The listing builds one solid part. Answer for the finished solid, in the listing's coordinates (mm). Face numbers are marked on the shaded views. A direction names the side the tool comes from. Coordinates: 2 decimals unless noted, no trailing zeros. Write each loop counter-clockwise with the first axis right and the second up, starting at its lowest first coordinate (ties: lowest second). Pieces come first, ordered by that corner, then holes.
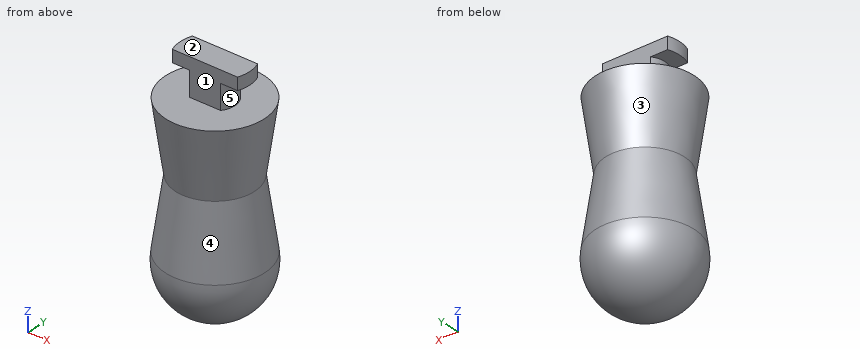
from build123d import *

# Parameters (mm, degrees)
F3_DEPTH = 9.525


with BuildPart() as f1:
    # F0 (on Front) → F1 (revolve)
    with BuildSketch(Plane.XZ):
        Polygon((0, -18.0305813839), (0, 0), (-5.08, 0), (-12.7, 0), (-10.16, -18.0305813839), align=None)
        Polygon((-5.08, 0), (0, 0), (0, 9.525), (-8.89, 9.525), (-8.89, 6.35), (-5.08, 6.35), align=None)
        Polygon((0, -36.0611627679), (0, -18.0305813839), (-10.16, -18.0305813839), (-12.7635, -36.0611627679), align=None)
        with BuildLine():
            Line((0, -50.8), (0, -36.0611627679))
            Line((0, -36.0611627679), (-12.7635, -36.0611627679))
            ThreePointArc((-12.7635, -36.0611627679), (-9.7485929139, -46.3461912692), (0, -50.8))
        make_face()
    revolve(axis=Axis((0, 0, -25.4), (0, 0, -1)))

    # F2 (on face) → F3 (cut, through all)
    with BuildSketch(Plane.XY.offset(9.525)):
        with BuildLine():
            ThreePointArc((8.3037024874, 3.175), (0, 8.89), (-8.3037024874, 3.175))
            Line((-8.3037024874, 3.175), (8.3037024874, 3.175))
        make_face()
        with BuildLine():
            Line((8.3037024874, -3.175), (-8.3037024874, -3.175))
            ThreePointArc((-8.3037024874, -3.175), (0, -8.89), (8.3037024874, -3.175))
        make_face()
        with BuildLine():
            ThreePointArc((10.9695693512, 3.175), (0, 11.4198107144), (-10.9695693512, 3.175))
            Line((-10.9695693512, 3.175), (-8.3037024874, 3.175))
            ThreePointArc((-8.3037024874, 3.175), (0, 8.89), (8.3037024874, 3.175))
            Line((8.3037024874, 3.175), (10.9695693512, 3.175))
        make_face()
        with BuildLine():
            Line((-8.3037024874, -3.175), (-10.9695693512, -3.175))
            ThreePointArc((-10.9695693512, -3.175), (0, -11.4198107144), (10.9695693512, -3.175))
            Line((10.9695693512, -3.175), (8.3037024874, -3.175))
            ThreePointArc((8.3037024874, -3.175), (0, -8.89), (-8.3037024874, -3.175))
        make_face()
        with BuildLine():
            Line((-8.3037024874, 3.175), (-10.9695693512, 3.175))
            ThreePointArc((-10.9695693512, 3.175), (-11.4198107144, 0), (-10.9695693512, -3.175))
            Line((-10.9695693512, -3.175), (-8.3037024874, -3.175))
            ThreePointArc((-8.3037024874, -3.175), (-8.89, 0), (-8.3037024874, 3.175))
        make_face()
        with BuildLine():
            ThreePointArc((11.4198107144, 0), (11.3066901072, 1.6033825405), (10.9695693512, 3.175))
            Line((10.9695693512, 3.175), (8.3037024874, 3.175))
            ThreePointArc((8.3037024874, 3.175), (8.7421969525, 1.6143396307), (8.89, 0))
            ThreePointArc((8.89, 0), (8.7421969525, -1.6143396307), (8.3037024874, -3.175))
            Line((8.3037024874, -3.175), (10.9695693512, -3.175))
            ThreePointArc((10.9695693512, -3.175), (11.3066901072, -1.6033825405), (11.4198107144, 0))
        make_face()
    extrude(amount=-F3_DEPTH, mode=Mode.SUBTRACT)


solid = f1.part
Q1. Which of the six approach directions +Z, -Z, +X, -X, +Y, -Y give full straight-line access (tool end or side, diameter ignored) to the marked faces 4 and 5?
Answers below:
face 4: none
face 5: +X
Q2. The part is cut by section D-D, the plane z = -32. Write down the section's boundary in (x, y).
Answers below:
outline: circle Ø24.35 at (0, 0)
Q3. The part is cut by section B-B, the plane x = 0. Write down the section's boundary in (y, z) (1 decimal).
Answers below:
outline: (-12.8, -36.1) arc R12.9 ccw (long way) to (12.8, -36.1) - (10.2, -18) - (12.7, 0) - (3.2, 0) - (3.2, 9.5) - (-3.2, 9.5) - (-3.2, 0) - (-12.7, 0) - (-10.2, -18) - close
Q4. Find the intervals of material crossed by probe 1 along Z at (x, y) = (7.5, 1.25) (3 decimals); probe 2 along Z at (x, y) = (-7.75, 3) (3 decimals); probe 3 along X at (y, z) = (11.5, -37), in increasing order.
Answers below:
probe 1: z = -48.32 to 0, 6.35 to 9.525
probe 2: z = -47.765 to 0, 6.35 to 9.525
probe 3: x = -5.77 to 5.77
Q5. The part is cut by section C-C, the plane z = 1.5. Write down the section's boundary in (x, y) (3 decimals).
Answers below:
outline: (-3.966, -3.175) - (3.966, -3.175) arc R5.08 ccw to (3.966, 3.175) - (-3.966, 3.175) arc R5.08 ccw to start
Q6. Determine the mould class of the marked faces 1, 2 and 3 for opening direction Z: released by +Z, released by -Z, zero draft, split by the parting line, or undercut.
Answers below:
face 1: zero draft
face 2: released by +Z
face 3: undercut
Q7. Given pin 1 (3 mm diameter, centred on x = -2.5, z = 3, fed in from +Y) (3 decimals); pin 2 (5.5 mm diameter, centred on x = -5.5, y = 1.5, fed in from -Z); pin 3 (3 mm diameter, centred on y = 6.5, z = -10, fed in from -X), each flat-ended and moving along its own axis, determine where each tip first touches the part or whether it passes through.
Answers below:
pin 1: stops at y = 3.175
pin 2: stops at z = -50.46
pin 3: stops at x = -10.16
